Geometry check sheet. Reference: drawing and pictorial views, mm from the part's lowest x, y, z. Give positions to 0.01 mm unless a question says otherwise; leave off trailing zeros. Write each loop counter-clockwise with the first axis right and the second up, starting at its lowest first coordinate (ties: lowest second). Pieces come first, ordered by that corner, then holes. Notation, with made-up numbers: M -29,76.5 L -10,76.5 A26 ccw -10,95.5 Z; hole C -6,66 d4. An arc over 180 degrees is marked long. One line per item, written item: value. Start each with the question number.
1. Cross-section at A-A on x = 5. Record the cut outline in (y, z).
2. Gauge pin test, flat ends, axial feed: pin 1 (4.5 mm diameter, centred on x = 5, y = 229, fed in from -Z); pin 2 (3.5 mm diameter, centred on x = 5, y = 50, fed in from -Z). Record the tip position at first contact, or that the pin passes through.
3. Cross-section at B-B on y = 8. Record the cut outline in (x, z), then the cut area to 3 significant figures.
4. Scan lines: line 1 (Y direction, x = 29, z = 1.7); line 2 (X direction, y = 229, z = 2.25); line 3 (X direction, y = 50.5, z = 2.7). Record each from-to range of solid material in increasing order.
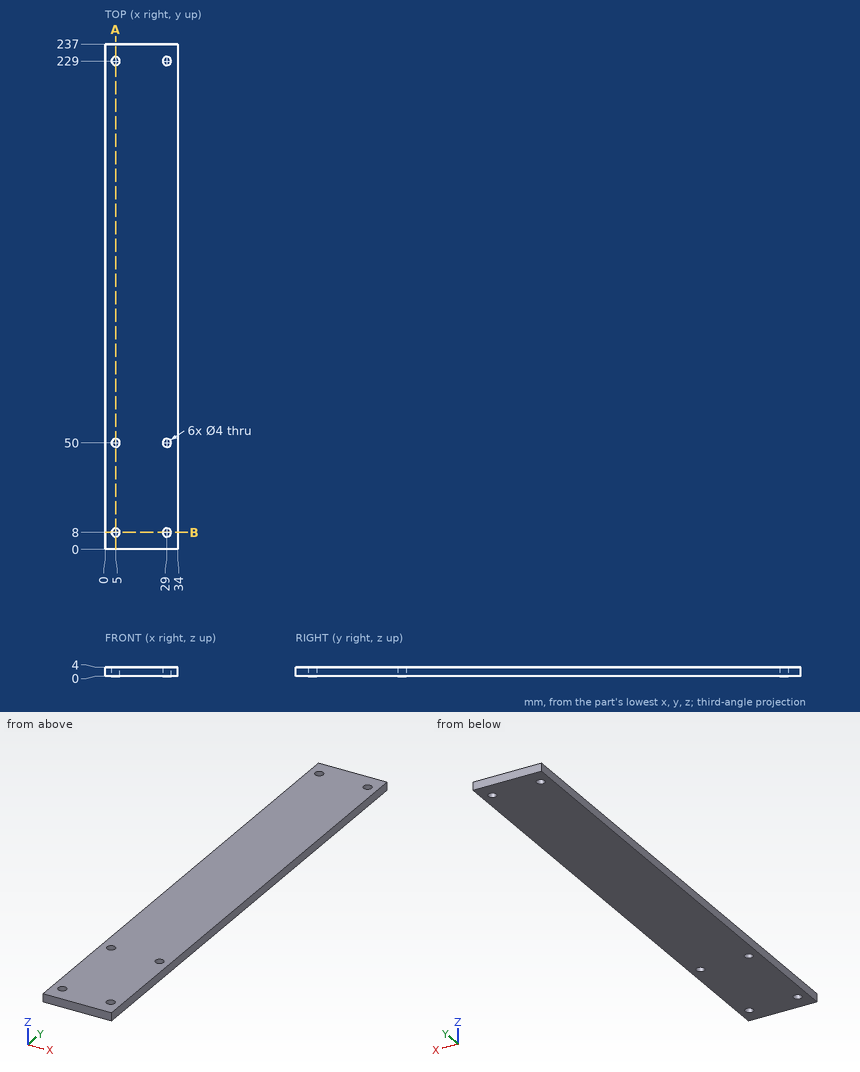
Report:
1. outline: M 0,0 L 6,0 L 6,4 L 0,4 Z; M 10,0 L 48,0 L 48,4 L 10,4 Z; M 52,0 L 227,0 L 227,4 L 52,4 Z; M 231,0 L 237,0 L 237,4 L 231,4 Z
2. pin 1: stops at z = 0
2. pin 2: passes through
3. outline: M 0,0 L 3,0 L 3,4 L 0,4 Z; M 7,0 L 27,0 L 27,4 L 7,4 Z; M 31,0 L 34,0 L 34,4 L 31,4 Z
3. area: 104 mm^2
4. line 1: y = 0 to 6, 10 to 48, 52 to 227, 231 to 237
4. line 2: x = 0 to 3, 7 to 27, 31 to 34
4. line 3: x = 0 to 3.06, 6.94 to 27.06, 30.94 to 34
